Here's how the part is built. I have some questions about the finished solid (model axes, mm). A direction names the side the tool comes from. Give positions to 0.01 mm unless a question says otherwise; leave off trailing zeros. Loops run counter-clockwise (first coordinate to the right, second up) from the corner with the lowest first, then second, coordinate; pieces in that order, holes last. Notation, with made-up numbers: (44, 57.5) - (98, 57.5) arc R26 cw to (98, 81.5) - close; hole circle Ø5 at (-35, 49). An arc over 180 degrees is marked (long way). Use one line per item in the form item = value.
from build123d import *

# Parameters (mm, degrees)
F2_R = 9
F3_R = 4


with BuildPart() as f1:
    # F0 (on Front) → F1 (revolve)
    with BuildSketch(Plane.XZ):
        Polygon((0, 1.822479), (0, 0), (64.008, 0), (64.008, 9.4996), (57.568784, 9.4996), (17.568784, 9.4996), (9.874334, 4.96087), (1.873334, 4.96087), (0, 4.2418), align=None)
    revolve(axis=Axis((32.004, 0, 0), (1, 0, 0)))

    # F2
    f2_edges = [f1.edges().sort_by_distance(p)[0] for p in [
        (64.008, 0, -9.4996),
    ]]
    fillet(f2_edges, radius=F2_R)

    # F3
    f3_edges = [f1.edges().sort_by_distance(p)[0] for p in [
        (17.568784, 0, -9.4996),
        (9.874334, 0, -4.96087),
        (1.873334, 0, -4.96087),
    ]]
    fillet(f3_edges, radius=F3_R)


solid = f1.part
(1) If we section it at B-B (x = 13.5): List the corners of the cut face in (y, z) for me, plus the area to 3 significant figures.
Geometry says:
outline = circle Ø14.2 at (0, 0)
area = 158 mm²
(2) For P1, Ø10, axis at x = 12, z = 6.5, coming from the +Y side; P2, Ø4, axis at x = 16, y = -5, coming from the -Z side; P3, Ø8, axis at x = 18, z = -4.5, coming from the -Y side, each with a flat end and sliding along its axis, tell me the tip position at first contact or that it passes through.
Geometry says:
P1 = 7.83
P2 = -8.58
P3 = -9.48
(3) For faces 1 (the cylindrical face through (5.66, -1.49, 4.73)), 2 (the flat face through (0, 0, 0)), which set-ups out of +Z, -Z, +X, -X, +Y, -Y let a thin tool reach every point of the face, with its end or its side?
Geometry says:
face_1 = -X
face_2 = +Z, -Z, -X, +Y, -Y
(4) If we section it at A-A (x = 24.5): List the corners of the cut face in (y, z) for me.
Geometry says:
outline = circle Ø19 at (0, 0)
(5) If I drill on probe 1 along Y at (x, z) = (41, -8.25); probe 2 along Y at (x, z) = (19, -8.5); probe 3 along Z at (x, y) = (47, -0.5), over which ranges is the centre line in solid material (lowest first)?
Geometry says:
probe_1 = -4.71 to 4.71
probe_2 = -4.24 to 4.24
probe_3 = -9.49 to 9.49
